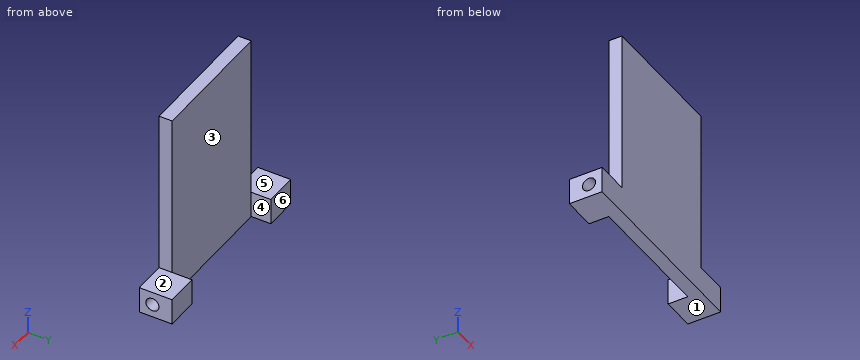
```python
from build123d import *

# Parameters (mm, degrees)
SKETCH5_W           = 100
SKETCH5_H           = 170
BOSS_EXTRUDE2_DEPTH = 10
SKETCH7_W           = 20
SKETCH7_H           = 25
BOSS_EXTRUDE3_DEPTH = 25
SKETCH8_W           = 20
SKETCH8_H           = 25
BOSS_EXTRUDE4_DEPTH = 25
SKETCH11_R          = 5
CUT_EXTRUDE1_DEPTH  = 20
CUT_EXTRUDE2_START  = -20
SKETCH12_R          = 5
CUT_EXTRUDE2_DEPTH  = 20
SKETCH17_W          = 100
SKETCH17_H          = 10
BOSS_EXTRUDE6_DEPTH = 100
SKETCH18_W          = 100
SKETCH18_H          = 125
CUT_EXTRUDE3_DEPTH  = 10


with BuildPart() as part:
    # Sketch5 → Boss-Extrude2 (new body)
    with BuildSketch(Plane(origin=(0, -50, 0), x_dir=(-1, 0, 0), z_dir=(0, -1, 0))):
        Rectangle(SKETCH5_W, SKETCH5_H)
    extrude(amount=-BOSS_EXTRUDE2_DEPTH)

    # Sketch7 → Boss-Extrude3 (add)
    with BuildSketch(Plane.ZY.offset(50)):
        with Locations((-75, -37.5)):
            Rectangle(SKETCH7_W, SKETCH7_H)
    extrude(amount=BOSS_EXTRUDE3_DEPTH)

    # Sketch8 → Boss-Extrude4 (add)
    with BuildSketch(Plane(origin=(50, 0, 0), x_dir=(0, 0, -1), z_dir=(1, 0, 0))):
        with Locations((75, -37.5)):
            Rectangle(SKETCH8_W, SKETCH8_H)
    extrude(amount=BOSS_EXTRUDE4_DEPTH)

    # Sketch11 → Cut-Extrude1 (cut)
    with BuildSketch(Plane.ZY.offset(75)):
        with Locations((-75, -40)):
            Circle(SKETCH11_R)
    extrude(amount=-CUT_EXTRUDE1_DEPTH, mode=Mode.SUBTRACT)

    # Sketch12 → Cut-Extrude2 (cut)
    with BuildSketch(Plane(origin=(75, 0, 0), x_dir=(0, 0, -1), z_dir=(1, 0, 0)).offset(CUT_EXTRUDE2_START)):
        with Locations(Location((75, -40, 0), (0, 0, 180))):
            Circle(SKETCH12_R)
    extrude(amount=CUT_EXTRUDE2_DEPTH, mode=Mode.SUBTRACT)

    # Sketch17 → Boss-Extrude6 (add)
    with BuildSketch(Plane.XY.offset(85)):
        with Locations((0, -45)):
            Rectangle(SKETCH17_W, SKETCH17_H)
    extrude(amount=BOSS_EXTRUDE6_DEPTH)

    # Sketch18 → Cut-Extrude3 (cut)
    with BuildSketch(Plane(origin=(0, -40, 0), x_dir=(1, 0, 0), z_dir=(0, 1, 0))):
        with Locations((0, -122.5)):
            Rectangle(SKETCH18_W, SKETCH18_H)
    extrude(amount=-CUT_EXTRUDE3_DEPTH, mode=Mode.SUBTRACT)


solid = part.part
```
Check sheet for the modelled part. Datum: model origin and axes. Units: mm. Face numbers are marked on the shaded views. A direction names the side the tool comes from. Round coordinates to 2 decimals unless told otherwise and drop trailing zeros. Loops run counter-clockwise (first coordinate to the right, second up) from the corner with the lowest first, then second, coordinate; pieces in that order, holes last. Notation, with made-up numbers: (11.25, 14.5) - (32.25, 14.5) arc R16 ccw to (32.25, 30.5) - close; hole circle Ø11 at (-12, 70.25). An arc over 180 degrees is marked (long way). Answer as a JSON object with one key per item and string values. Group by question number.
Q1. Scan lines: line 1 along Y through (x, z) = (71, -75); line 2 along Z through (x, y) = (65.25, -40); line 3 along X through (y, z) = (-46, -20). Record each from-to range of solid material in increasing order. Write a range as [from, to].
Q2. Mould release check, pull along Z, two halves, no side actions. Record for the marked faces 1, 2 and 3: released by +Z, released by -Z, zero draft, split by the parting line, or undercut.
Q3. Sectioned sample at B-B, the plane x = -61.5. Enter the section's corners in (y, z), plus the area to 3 significant figures.
Q4. Gauge pin test, flat ends, axial feed: P1, Ø3, axis at y = -46, z = -33, coming from the -X side; P2, Ø3, axis at y = -40, z = -77, coming from the -X side; P3, Ø12, axis at x = 23, z = -6.5, coming from the +Y side. Record the tip position at first contact, or that the pin passes through.
Q5. Sectioned sample at A-A, the plane y = -32.75. Enter the section's corners in (x, z).
Q6. Sectioned sample at D-D, the plane x = 12. Enter the section's corners in (y, z), plus the area to 3 significant figures.
Q7. Set-up check for the marked faces 4, 5 and 6: record each of +Z, -Z, +X, -X, +Y, -Y from which the full face is reachable in a straight line by a thin tool's end or side.
Q8. Sectioned sample at C-C, the plane z = -75. Enter the section's corners in (x, y), plus the area to 3 significant figures.
Solution:
{
 "1": {"line 1": "y = [-50, -45], [-35, -25]", "line 2": "z = [-85, -80], [-70, -65]", "line 3": "x = [-50, 50]"},
 "2": {"face 1": "released by -Z", "face 2": "released by +Z", "face 3": "zero draft"},
 "3": {"outline": "(-50, -85) - (-25, -85) - (-25, -65) - (-50, -65) - close; hole circle Ø10 at (-40, -75)", "area": "421 mm²"},
 "4": {"P1": "stops at x = -50", "P2": "stops at x = -55", "P3": "stops at y = -40"},
 "5": {"outline": "(-75, -85) - (-50, -85) - (-50, -65) - (-75, -65) - close; (50, -85) - (75, -85) - (75, -65) - (50, -65) - close"},
 "6": {"outline": "(-50, -85) - (-40, -85) - (-40, 60) - (-50, 60) - close", "area": "1,450 mm²"},
 "7": {"face 4": "+Z, -Z, +Y", "face 5": "+Z, -X, +Y, -Y", "face 6": "+Z, -Z, +X, -X, +Y"},
 "8": {"outline": "(-75, -50) - (75, -50) - (75, -45) - (55, -45) - (55, -35) - (75, -35) - (75, -25) - (50, -25) - (50, -40) - (-50, -40) - (-50, -25) - (-75, -25) - (-75, -35) - (-55, -35) - (-55, -45) - (-75, -45) - close", "area": "1,850 mm²"}
}
